Verification items for the finished model (mm, model axes). Face numbers are marked on the shaded views. A direction names the side the tool comes from. Give positions to 0.01 mm unless a question says otherwise; leave off trailing zeros. Loops run counter-clockwise (first coordinate to the right, second up) from the corner with the lowest first, then second, coordinate; pieces in that order, holes last. Notation, with made-up numbers: M 57,2.5 L 98,2.5 A36 ccw 98,36.5 Z; hole C 67,-38 d6. An arc over 180 degrees is marked long. Use a Markdown table: item, result.
Autodesk Fusion 360 part; units mm, degrees
sketch "Sketch1" plane through (0, 0, 0) normal (0, 0, 1) x (1, 0, 0)
  line L0 (0, 0) -> (110, 0)
  line L1 (110, 0) -> (110, 20)
  line L2 (110, 20) -> (0, 20)
  line L3 (0, 20) -> (0, 0)
  dimension "d1" = 110
  dimension "d2" = 20
extrude "Extrude1" add sketch "Sketch1" along normal blind 5
sketch "Sketch2" plane through (0, 0, 5) normal (0, 0, 1) x (-1, 0, 0)
  line L0 (0, -20) -> (0, 0)
  line L1 (0, 0) -> (-110, 0)
  line L2 (-110, 0) -> (-110, -20)
  line L3 (-110, -20) -> (0, -20)
  line L4 (-3.85, -2) -> (-106.15, -2) construction
  line L5 (-46, -2) -> (-46, -6.5) construction
  line L6 (-91.95, -6.5) -> (-91.95, -2)
  line L7 (-97.15, -6.5) -> (-91.95, -6.5)
  line L8 (-73.95, -6.5) -> (-73.95, -2)
  line L9 (-55, -2) -> (-55, -6.5) construction
  line L10 (-33.45, -2) -> (-33.45, -6.5) construction
  line L11 (-27.05, -2) -> (-27.05, -6.5)
  line L12 (-30.85, -6.5) -> (-30.85, -2)
  line L13 (-43.4, -6.5) -> (-43.4, -2)
  line L14 (-18.05, -2) -> (-18.05, -6.5)
  line L15 (-21.85, -6.5) -> (-21.85, -2)
  line L16 (-36.05, -6.5) -> (-30.85, -6.5)
  line L17 (-9.05, -2) -> (-9.05, -6.5)
  line L18 (-9.05, -6.5) -> (-3.85, -6.5)
  line L19 (-21.85, -2) -> (-27.05, -2)
  line L20 (-3.85, -2) -> (-9.05, -2)
  line L21 (-12.85, -2) -> (-18.05, -2)
  line L22 (-3.85, -6.5) -> (-3.85, -2)
  line L23 (-18.05, -6.5) -> (-12.85, -6.5)
  line L24 (-30.85, -2) -> (-36.05, -2)
  line L25 (-82.95, -6.5) -> (-82.95, -2)
  line L26 (-57.6, -2) -> (-57.6, -6.5)
  line L27 (-48.6, -2) -> (-48.6, -6.5)
  line L28 (-61.4, -2) -> (-66.6, -2)
  line L29 (-64, -2) -> (-64, -6.5) construction
  line L30 (-106.15, -6.5) -> (-100.95, -6.5)
  line L31 (-100.95, -2) -> (-106.15, -2)
  line L32 (-106.15, -2) -> (-106.15, -6.5)
  line L33 (-79.15, -2) -> (-79.15, -6.5)
  line L34 (-61.4, -6.5) -> (-61.4, -2)
  line L35 (-52.4, -6.5) -> (-52.4, -2)
  line L36 (-88.15, -6.5) -> (-82.95, -6.5)
  line L37 (-97.15, -2) -> (-97.15, -6.5)
  line L38 (-106.15, -2) -> (-106.15, -6.5) construction
  line L39 (-48.6, -6.5) -> (-43.4, -6.5)
  line L40 (-52.4, -2) -> (-57.6, -2)
  line L41 (-76.55, -2) -> (-76.55, -6.5) construction
  line L42 (-43.4, -2) -> (-48.6, -2)
  line L43 (-57.6, -6.5) -> (-52.4, -6.5)
  line L44 (-66.6, -6.5) -> (-61.4, -6.5)
  line L45 (-82.95, -2) -> (-88.15, -2)
  line L46 (-66.6, -2) -> (-66.6, -6.5)
  line L47 (-100.95, -6.5) -> (-100.95, -2)
  line L48 (-91.95, -2) -> (-97.15, -2)
  line L49 (-88.15, -2) -> (-88.15, -6.5)
  line L50 (-27.05, -6.5) -> (-21.85, -6.5)
  line L51 (-12.85, -6.5) -> (-12.85, -2)
  line L52 (-36.05, -2) -> (-36.05, -6.5)
  line L53 (-3.85, -6.5) -> (-3.85, -2) construction
  line L54 (-73.95, -2) -> (-79.15, -2)
  line L55 (-106.15, -6.5) -> (-3.85, -6.5) construction
  line L56 (-79.15, -6.5) -> (-73.95, -6.5)
  line L57 (0, -2) -> (-110, -2) construction
  line L58 (-55, -20) -> (-55, 0) construction
  dimension "d27" = 9
  dimension "d28" = 0
  dimension "d31" = 9
  dimension "d32" = 0
  dimension "d35" = 9
  dimension "d36" = 0
  dimension "d37" = 5.2
  dimension "d38" = 4.5
  dimension "d39" = 5.2
  dimension "d40" = 4.5
  dimension "d41" = 12.55
  dimension "d42" = 5.2
  dimension "d43" = 4.5
  dimension "d44" = 12.55
  dimension "d45" = 2
extrude "Extrude2" cut sketch "Sketch2" against normal blind 4 contours L6 L7 L37 L48 | L8 L33 L54 L56 | L11 L15 L19 L50 | L12 L16 L24 L52 | L13 L27 L39 L42 | L14 L21 L23 L51 | L17 L18 L20 L22 | L25 L36 L45 L49 | L26 L35 L40 L43 | L28 L34 L44 L46 | L30 L31 L32 L47
sketch "Sketch3" plane through (0, 0, 1) normal (0, 0, 1) x (-1, 0, 0)
  line L0 (-3.85, -6.5) -> (-3.85, -2)
  line L1 (-3.85, -2) -> (-9.05, -2)
  line L2 (-9.05, -2) -> (-9.05, -6.5)
  line L3 (-9.05, -6.5) -> (-3.85, -6.5)
  line L4 (-4.35, -6) -> (-8.55, -6)
  line L5 (-8.55, -6) -> (-8.55, -2.5)
  line L6 (-8.55, -2.5) -> (-4.35, -2.5)
  line L7 (-4.35, -2.5) -> (-4.35, -6)
  line L8 (-13.35, -6) -> (-17.55, -6)
  line L9 (-17.55, -6) -> (-17.55, -2.5)
  line L10 (-17.55, -2.5) -> (-13.35, -2.5)
  line L11 (-13.35, -2.5) -> (-13.35, -6)
  line L12 (-22.35, -6) -> (-26.55, -6)
  line L13 (-26.55, -6) -> (-26.55, -2.5)
  line L14 (-26.55, -2.5) -> (-22.35, -2.5)
  line L15 (-22.35, -2.5) -> (-22.35, -6)
  line L16 (-31.35, -6) -> (-35.55, -6)
  line L17 (-35.55, -6) -> (-35.55, -2.5)
  line L18 (-35.55, -2.5) -> (-31.35, -2.5)
  line L19 (-31.35, -2.5) -> (-31.35, -6)
  line L20 (-43.9, -6) -> (-48.1, -6)
  line L21 (-48.1, -6) -> (-48.1, -2.5)
  line L22 (-48.1, -2.5) -> (-43.9, -2.5)
  line L23 (-43.9, -2.5) -> (-43.9, -6)
  line L24 (-43.4, -6.5) -> (-48.6, -6.5)
  line L25 (-48.6, -2) -> (-43.4, -2)
  line L26 (-48.6, -6.5) -> (-48.6, -2)
  line L27 (-43.4, -2) -> (-43.4, -6.5)
  line L28 (-52.9, -6) -> (-57.1, -6)
  line L29 (-57.1, -6) -> (-57.1, -2.5)
  line L30 (-57.1, -2.5) -> (-52.9, -2.5)
  line L31 (-52.9, -2.5) -> (-52.9, -6)
  line L32 (-61.9, -6) -> (-66.1, -6)
  line L33 (-66.1, -6) -> (-66.1, -2.5)
  line L34 (-66.1, -2.5) -> (-61.9, -2.5)
  line L35 (-61.9, -2.5) -> (-61.9, -6)
  line L36 (-78.65, -2.5) -> (-74.45, -2.5)
  line L37 (-78.65, -6) -> (-78.65, -2.5)
  line L38 (-74.45, -6) -> (-78.65, -6)
  line L39 (-74.45, -2.5) -> (-74.45, -6)
  line L40 (-73.95, -6.5) -> (-79.15, -6.5)
  line L41 (-79.15, -2) -> (-73.95, -2)
  line L42 (-79.15, -6.5) -> (-79.15, -2)
  line L43 (-73.95, -2) -> (-73.95, -6.5)
  line L44 (-87.65, -6) -> (-87.65, -2.5)
  line L45 (-87.65, -2.5) -> (-83.45, -2.5)
  line L46 (-83.45, -2.5) -> (-83.45, -6)
  line L47 (-83.45, -6) -> (-87.65, -6)
  line L48 (-96.65, -6) -> (-96.65, -2.5)
  line L49 (-96.65, -2.5) -> (-92.45, -2.5)
  line L50 (-92.45, -2.5) -> (-92.45, -6)
  line L51 (-92.45, -6) -> (-96.65, -6)
  line L52 (-105.65, -6) -> (-105.65, -2.5)
  line L53 (-105.65, -2.5) -> (-101.45, -2.5)
  line L54 (-101.45, -2.5) -> (-101.45, -6)
  line L55 (-101.45, -6) -> (-105.65, -6)
  dimension "d48" = 0.5
  dimension "d49" = 0.5
  dimension "d50" = 0.5
  dimension "d51" = 0.5
  dimension "d54" = -9
  dimension "d55" = 0
  dimension "d56" = 0.5
  dimension "d57" = 0.5
  dimension "d58" = 0.5
  dimension "d59" = 0.5
  dimension "d62" = -9
  dimension "d63" = 0
  dimension "d64" = 0.5
  dimension "d65" = 0.5
  dimension "d66" = 0.5
  dimension "d67" = 0.5
  dimension "d70" = -9
  dimension "d71" = 0
extrude "Extrude3" cut sketch "Sketch3" against normal blind 2 contours L4 L5 L6 L7 | L8 L9 L10 L11 | L12 L13 L14 L15 | L16 L17 L18 L19 | L20 L21 L22 L23 | L28 L29 L30 L31 | L32 L33 L34 L35 | L36 L37 L38 L39 | L44 L45 L46 L47 | L48 L49 L50 L51 | L52 L53 L54 L55
sketch "Sketch4" plane through (0, 0, 5) normal (0, 0, 1) x (-1, 0, 0)
  line L0 (0, -20) -> (0, 0)
  line L1 (0, 0) -> (-110, 0)
  line L2 (-110, 0) -> (-110, -20)
  line L3 (-110, -20) -> (0, -20)
  line L4 (-106.15, -2) -> (-100.95, -2)
  line L5 (-100.95, -2) -> (-100.95, -6.5)
  line L6 (-100.95, -6.5) -> (-106.15, -6.5)
  line L7 (-106.15, -6.5) -> (-106.15, -2)
  line L8 (-61.4, -6.5) -> (-66.6, -6.5)
  line L9 (-66.6, -6.5) -> (-66.6, -2)
  line L10 (-66.6, -2) -> (-61.4, -2)
  line L11 (-61.4, -2) -> (-61.4, -6.5)
  line L12 (-21.85, -2) -> (-21.85, -6.5)
  line L13 (-21.85, -6.5) -> (-27.05, -6.5)
  line L14 (-27.05, -6.5) -> (-27.05, -2)
  line L15 (-27.05, -2) -> (-21.85, -2)
  line L16 (-18.05, -2) -> (-12.85, -2)
  line L17 (-12.85, -2) -> (-12.85, -6.5)
  line L18 (-12.85, -6.5) -> (-18.05, -6.5)
  line L19 (-18.05, -6.5) -> (-18.05, -2)
  line L20 (-52.4, -2) -> (-52.4, -6.5)
  line L21 (-52.4, -6.5) -> (-57.6, -6.5)
  line L22 (-57.6, -6.5) -> (-57.6, -2)
  line L23 (-57.6, -2) -> (-52.4, -2)
  line L24 (-97.15, -6.5) -> (-97.15, -2)
  line L25 (-97.15, -2) -> (-91.95, -2)
  line L26 (-91.95, -2) -> (-91.95, -6.5)
  line L27 (-91.95, -6.5) -> (-97.15, -6.5)
  line L28 (-73.95, -2) -> (-73.95, -6.5)
  line L29 (-73.95, -6.5) -> (-79.15, -6.5)
  line L30 (-79.15, -6.5) -> (-79.15, -2)
  line L31 (-79.15, -2) -> (-73.95, -2)
  line L32 (-30.85, -6.5) -> (-36.05, -6.5)
  line L33 (-36.05, -6.5) -> (-36.05, -2)
  line L34 (-36.05, -2) -> (-30.85, -2)
  line L35 (-30.85, -2) -> (-30.85, -6.5)
  line L36 (-9.05, -2) -> (-3.85, -2)
  line L37 (-3.85, -2) -> (-3.85, -6.5)
  line L38 (-3.85, -6.5) -> (-9.05, -6.5)
  line L39 (-9.05, -6.5) -> (-9.05, -2)
  line L40 (-48.6, -6.5) -> (-48.6, -2)
  line L41 (-48.6, -2) -> (-43.4, -2)
  line L42 (-43.4, -2) -> (-43.4, -6.5)
  line L43 (-43.4, -6.5) -> (-48.6, -6.5)
  line L44 (-82.95, -6.5) -> (-88.15, -6.5)
  line L45 (-88.15, -6.5) -> (-88.15, -2)
  line L46 (-88.15, -2) -> (-82.95, -2)
  line L47 (-82.95, -2) -> (-82.95, -6.5)
  line L48 (-21.85, -6.5) -> (-18.05, -6.5) construction
  line L49 (-19.95, -6.5) -> (-19.95, -20) construction
  line L50 (-88.15, -6.5) -> (-91.95, -6.5) construction
  line L51 (-90.05, -6.5) -> (-90.05, -20) construction
  circle A0 centre (-19.95, -13.25) radius 4.5
  circle A1 centre (-90.05, -13.25) radius 4.5
  line L52 (-19.95, -17.75) -> (-90.05, -17.75)
  line L53 (-90.05, -8.75) -> (-19.95, -8.75)
  dimension "d80" = 9
  dimension "d81" = 9
extrude "Extrude4" cut sketch "Sketch4" against normal blind 5 contours A0 | A0 A1 L52 L53 | A1
chamfer "Chamfer1" distance 1 angle 60 4 edges at (55, 20, 5) (0, 10, 5) (55, 0, 5) (110, 10, 5) measured on face at (101.8291, 13.3621, 5) measured on face at (101.8291, 13.3621, 5) measured on face at (101.8291, 13.3621, 5) measured on face at (101.8291, 13.3621, 5)
equation "d37 = 5 mm + 0.2 mm"
equation "d38 = 4.3 mm + 0.2 mm"
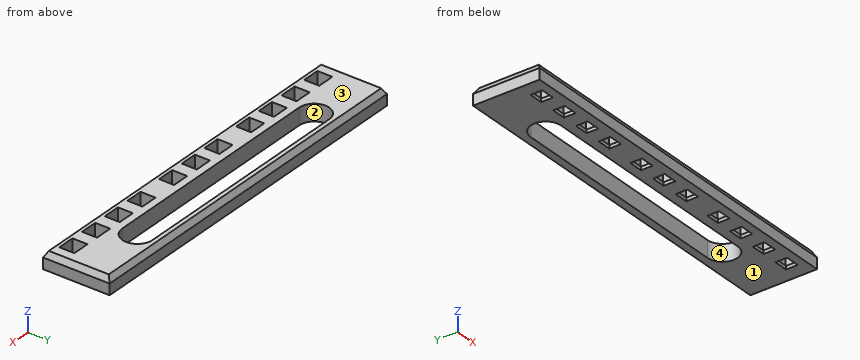
(1) Cross-section at A-A on y = 13.25. Record the cut outline in (x, z).
Results below:
| item | result |
|---|---|
| outline | M 0,0 L 15.45,0 L 15.45,5 L 1,5 L 0,3.27 Z; M 94.55,0 L 110,0 L 110,3.27 L 109,5 L 94.55,5 Z |
(2) Material ranges on line 1 (Y direction, x = 65, z = 0.35); line 2 (Y direction, x = 56, z = 1.35); line 3 (Y direction, x = 90.5, z = 1.35), recorded low to high.
Results below:
| item | result |
|---|---|
| line 1 | 0 to 2.5, 6 to 8.75, 17.75 to 20 |
| line 2 | 0 to 2, 6.5 to 8.75, 17.75 to 20 |
| line 3 | 0 to 8.77, 17.73 to 20 |
(3) Draft check along Y on the marked faces 1 and 2. Enter one of: +Y half, -Y half, draft (parallel to the pull), parting line (faces both ways), or undercut.
Results below:
| item | result |
|---|---|
| face 1 | draft |
| face 2 | undercut |
(4) Cross-section at B-B on y = 3.75. State how many separate pieces and enclosed holes the cut face has, then the cut area to 3 significant figures.
Results below:
| item | result |
|---|---|
| separate pieces | 12 |
| enclosed holes | 0 |
| area | 273 mm^2 |
(5) Set-up check for the marked faces 3 and 4: record each of +Z, -Z, +X, -X, +Y, -Y from which the full face is reachable in a straight line by a thin tool's end or side.
Results below:
| item | result |
|---|---|
| face 3 | +Z, +X, -X, +Y, -Y |
| face 4 | +Z, -Z |
